```python
from build123d import *

# Parameters (mm, degrees)
BOSS_EXTRUDE1_DEPTH = 40
FILLET1_R           = 20
BOSS_EXTRUDE2_DEPTH = 10
CUT_EXTRUDE1_DEPTH  = 6
BOSS_EXTRUDE3_DEPTH = 10
CUT_EXTRUDE3_DEPTH  = 6
SKETCH15_R          = 15
SKETCH15_R_2        = 11
BOSS_EXTRUDE4_DEPTH = 18
CUT_EXTRUDE4_START  = -7
SKETCH16_R          = 11
CUT_EXTRUDE4_DEPTH  = 7


with BuildPart() as part:
    # Sketch1 → Boss-Extrude1 (new body)
    with BuildSketch(Plane.XY):
        Polygon((0, 0), (-32, 0), (-32, 7), (-7, 7), (-7, 70), (0, 70), align=None)
    extrude(amount=-BOSS_EXTRUDE1_DEPTH)

    # Fillet1
    fillet1_edges = [part.edges().sort_by_distance(p)[0] for p in [
        (-3.5, 70, 0),
        (-3.5, 70, -40),
    ]]
    fillet(fillet1_edges, radius=FILLET1_R - 0.0001)  # a hair under: the kernel refuses the full size

    # Sketch7 → Boss-Extrude2 (add)
    with BuildSketch(Plane.XY):
        Polygon((-7, 7), (-27, 7), (-7, 27), align=None)
    extrude(amount=-BOSS_EXTRUDE2_DEPTH)

    # Sketch11 → Cut-Extrude1 (cut)
    with BuildSketch(Plane.XY):
        Polygon((-7, 27), (-7, 7), (-27, 7), align=None)
    extrude(amount=-CUT_EXTRUDE1_DEPTH, mode=Mode.SUBTRACT)

    # Sketch12 → Boss-Extrude3 (add)
    with BuildSketch(Plane(origin=(0, 0, -40), x_dir=(-1, 0, 0), z_dir=(0, 0, -1))):
        Polygon((7, 27), (7, 7), (27, 7), align=None)
    extrude(amount=-BOSS_EXTRUDE3_DEPTH)

    # Sketch13 → Cut-Extrude3 (cut)
    with BuildSketch(Plane(origin=(0, 0, -40), x_dir=(-1, 0, 0), z_dir=(0, 0, -1))):
        Polygon((7, 27), (27, 7), (7, 7), align=None)
    extrude(amount=-CUT_EXTRUDE3_DEPTH, mode=Mode.SUBTRACT)

    # Sketch15 → Boss-Extrude4 (add)
    with BuildSketch(Plane.ZY.offset(7)):
        with Locations(Location((-20, 50, 0), (0, 0, 270))):
            Circle(SKETCH15_R)
        with Locations(Location((-20, 50, 0), (0, 0, 270))):
            Circle(SKETCH15_R_2, mode=Mode.SUBTRACT)
    extrude(amount=BOSS_EXTRUDE4_DEPTH)

    # Sketch16 → Cut-Extrude4 (cut)
    with BuildSketch(Plane.ZY.offset(7).offset(CUT_EXTRUDE4_START)):
        with Locations(Location((-20, 50, 0), (0, 0, 270))):
            Circle(SKETCH16_R)
    extrude(amount=CUT_EXTRUDE4_DEPTH, mode=Mode.SUBTRACT)


solid = part.part
```
CAD build for the part. Positions are in the model's coordinates, mm. A direction names the side the tool comes from. Round coordinates to 2 decimals unless told otherwise and drop trailing zeros. Order: outer loops, then holes, each group sorted by start corner. A loop starts at its lowest first (then second) coordinate and runs counter-clockwise, first axis right, second up. Notation, with made-up numbers: (-28, -28.5) - (18, -28.5) arc R25 ccw to (18, 3.5) - close; hole circle Ø7 at (8, 85). An arc over 180 degrees is marked (long way). Answer as CSV lines item,"result". Start each with the question number.
1. Saw through at C-C, the plane y = 43.5. Write the cut outline in (x, z).
2. Pull direction Z, two halves, no side cores. Call faces 1 (the face through (-16, 0, -20)), 2 (the face through (-3.451, 64.297, -33.986)), 3 (the face through (-20, 7, -20)): +Z half, -Z half, draft (parallel to the pull), parting line (faces both ways), or undercut.
3. Saw through at D-D, the plane y = 13.5. Write the cut outline in (x, z), and give its area (3 significant figures).
4. Tool access for faces 4 (the face through (-12, 13, -10)), 5 (the face through (-17, 17, -32)), 6 (the face through (-12, 13, -6)), 7 (the face through (-25, 55, -10)), 8 (the face through (-13, 13, -34)): list every direction of +Z, -Z, +X, -X, +Y, -Y with a clear straight run to the whole face (end or side of a thin tool).
5. Saw through at B-B, the plane z = -11.5. Write the cut outline in (x, y), and give its area (3 significant figures).
6. Drill centre lines: L1, parallel to Z at x = -15, y = 50; L2, parallel to Z at x = -14, y = 10.5; L3, parallel to Y at x = -16, z = -17. Where is each one in solid material? Low to high. Write a range as [from, to].
7. Pin check, flat tips, straight feed: pin 1 (2 mm diameter, centred on x = -11.5, y = 37, fed in from +Z); pin 2 (12.5 mm diameter, centred on x = -23, z = -22, fed in from +Y); pin 3 (5 mm diameter, centred on x = -24, z = -9, fed in from +Y). Stop position of each tip, or through.
Model answer:
1,outline,"(-25, -33.52) - (-7, -33.52) - (-7, -40) - (0, -40) - (0, -28.87) - (-25, -28.87) - close; (-25, -11.13) - (0, -11.13) - (0, 0) - (-7, 0) - (-7, -6.48) - (-25, -6.48) - close"
2,face 1,"draft"
2,face 2,"-Z half"
2,face 3,"undercut"
3,outline,"(-20.5, -34) - (-7, -34) - (-7, -40) - (0, -40) - (0, 0) - (-7, 0) - (-7, -6) - (-20.5, -6) - (-20.5, -10) - (-7, -10) - (-7, -30) - (-20.5, -30) - close"
3,area,"388 mm²"
4,face 4,"-X"
4,face 5,"+Z, -Z, -X"
4,face 6,"+Z, -X"
4,face 7,"+Z, -Z, -X, +Y"
4,face 8,"-Z, -X"
5,outline,"(-32, 0) - (0, 0) - (0, 43.02) - (-25, 43.02) - (-25, 37.64) - (-7, 37.64) - (-7, 7) - (-32, 7) - close; (-25, 56.98) - (0, 56.98) - (0, 68.1) - (-7, 68.1) - (-7, 62.36) - (-25, 62.36) - close"
5,area,"748 mm²"
6,L1,"z = [-35, -31], [-9, -5]"
6,L2,"z = [-34, -30], [-10, -6]"
6,L3,"y = [0, 7], [35.3, 39.42], [60.58, 64.7]"
7,pin 1,"stops at z = -11"
7,pin 2,"stops at y = 65"
7,pin 3,"stops at y = 62.36"
